Verification items for the finished model (mm, model axes). Face numbers are marked on the shaded views. A direction names the side the tool comes from. Coordinates: 2 decimals unless noted, no trailing zeros. Loops run counter-clockwise (first coordinate to the right, second up) from the corner with the lowest first, then second, coordinate; pieces in that order, holes last. Notation, with made-up numbers: (-15.5, 79) - (-7.5, 79) arc R23 cw to (-7.5, 96) - close; hole circle Ø5 at (82.25, 88.25). An arc over 180 degrees is marked (long way). One line per item, written item: value. Start each with the question number.
(1) Section check C-C (z = 4). Record the boundary of the cut face in (x, y).
(2) Section check B-B (x = 0). Record the boundary of the cut face in (y, z), plus the area to 3 significant figures.
(3) Section check D-D (x = -4). Record the boundary of the cut face in (y, z), plus the area to 3 significant figures.
(4) Gauge pin test, flat ends, axial feed: P1, Ø2.5, axis at y = 1, z = 10.5, coming from the +X side; P2, Ø2, axis at x = -3.5, y = 2.5, coming from the +Z side; P3, Ø3, axis at y = 1, z = 3.5, coming from the -X side. Record the tip position at first contact, or that the pin passes through.
(5) Section check A-A (y = 0). Record the boundary of the cut face in (x, z), plus the area to 3 significant figures.
(6) Set-up check for the marked faces 1, 2 and 3: record each of +Z, -Z, +X, -X, +Y, -Y from which the full face is reachable in a straight line by a thin tool's end or side.
(7) Thickness scan on probe 1 along Z at (x, y) = (4.25, -3.75); probe 2 along Z at (x, y) = (2.5, -0.75); probe 3 along Y at (x, z) = (-1.5, 6.5). Record the ranges inside material, lowest first. Write a range as [from, to].
```python
from build123d import *

# Parameters (mm, degrees)
SKETCH_W     = 9.7
SKETCH_H     = 11
PAD_DEPTH    = 6.8
SKETCH001_R  = 3.4
PAD001_DEPTH = 4.5
SKETCH002_R  = 3
PAD002_DEPTH = 13.5
SKETCH003_W  = 1.5
SKETCH003_H  = 5
POCKET_DEPTH = 3
CHAMFER_SIZE = 0.5


with BuildPart() as part:
    # Sketch → Pad (new body)
    with BuildSketch(Plane.XY):
        Rectangle(SKETCH_W, SKETCH_H)
    extrude(amount=-PAD_DEPTH)

    # Sketch001 → Pad001 (join)
    with BuildSketch(Plane.XY):
        Circle(SKETCH001_R)
    extrude(amount=PAD001_DEPTH)

    # Sketch002 → Pad002 (join)
    with BuildSketch(Plane.XY):
        Circle(SKETCH002_R)
    extrude(amount=PAD002_DEPTH)

    # Sketch003 → Pocket (cut, symmetric)
    with BuildSketch(Plane.XZ):
        with Locations((2.25, 11)):
            Rectangle(SKETCH003_W, SKETCH003_H)
    extrude(amount=POCKET_DEPTH, both=True, mode=Mode.SUBTRACT)

    # Chamfer
    chamfer_edges = [part.edges().sort_by_distance(p)[0] for p in [
        (-3, 0, 13.5),
    ]]
    chamfer(chamfer_edges, length=CHAMFER_SIZE)


solid = part.part
```
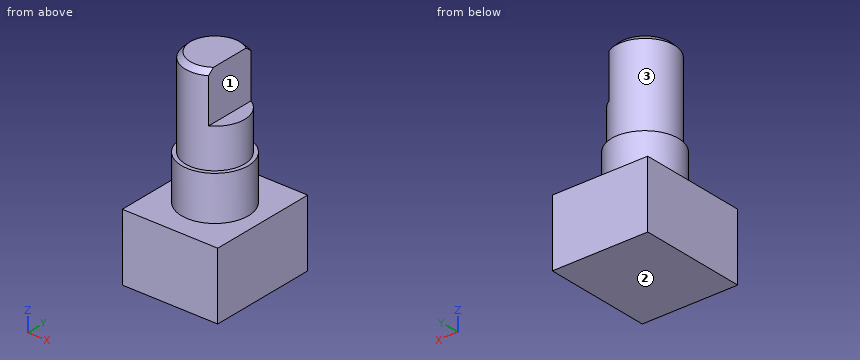
Responses:
1. outline: circle Ø6.8 at (0, 0)
2. outline: (-5.5, -6.8) - (5.5, -6.8) - (5.5, 0) - (3.4, 0) - (3.4, 4.5) - (3, 4.5) - (3, 13) - (2.5, 13.5) - (-2.5, 13.5) - (-3, 13) - (-3, 4.5) - (-3.4, 4.5) - (-3.4, 0) - (-5.5, 0) - close
2. area: 159 mm²
3. outline: (-5.5, -6.8) - (5.5, -6.8) - (5.5, 0) - (-5.5, 0) - close
3. area: 74.8 mm²
4. P1: stops at x = 1.5
4. P2: stops at z = 4.5
4. P3: stops at x = -3.4
5. outline: (-4.85, -6.8) - (4.85, -6.8) - (4.85, 0) - (3.4, 0) - (3.4, 4.5) - (3, 4.5) - (3, 8.5) - (1.5, 8.5) - (1.5, 13.5) - (-2.5, 13.5) - (-3, 13) - (-3, 4.5) - (-3.4, 4.5) - (-3.4, 0) - (-4.85, 0) - close
5. area: 143 mm²
6. face 1: +Z, +X, +Y, -Y
6. face 2: -Z, +X, -X, +Y, -Y
6. face 3: +Z
7. probe 1: z = [-6.8, 0]
7. probe 2: z = [-6.8, 8.5]
7. probe 3: y = [-2.6, 2.6]
